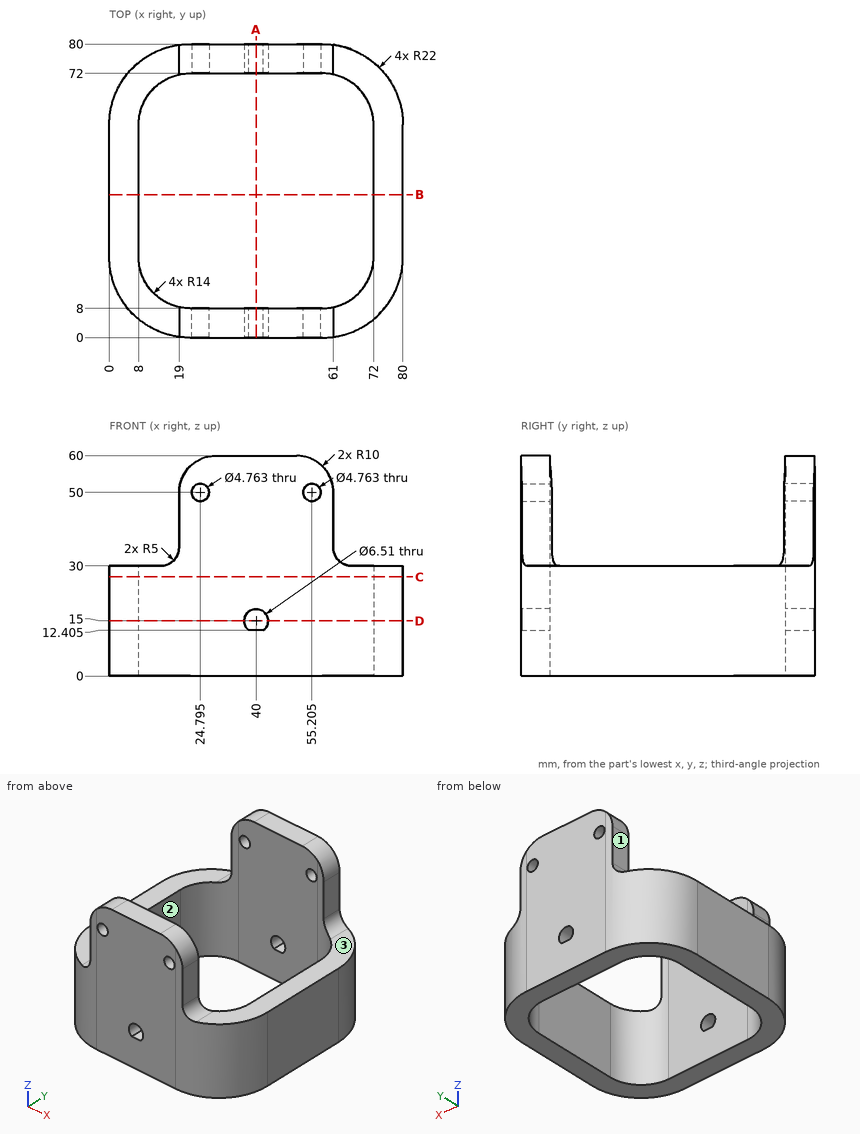
Check sheet for the drawn part. Datum: minimum x, y, z corner. Units: mm. A direction names the side the tool comes from. Coordinates: 2 decimals unless noted, no trailing zeros. Order: outer loops, then holes, each group sorted by start corner. A loop starts at its lowest first (then second) coordinate and runs counter-clockwise, first axis right, second up. Notation, with made-up numbers: (14.5, 77.25) - (23.5, 77.25) arc R5 cw to (23.5, 82.25) - close; hole circle Ø11 at (13.5, 8.25). An arc over 180 degrees is marked (long way). Return JSON: item names as keys, results as strings.
(1) Go/stop test with flat-tipped pins: pin 1 (2.5 mm diameter, centred on y = 75, z = 41, fed in from +X); pin 2 (11 mm diameter, centred on x = 9.5, y = 32, fed in from +Z); pin 3 (3 mm diameter, centred on y = 14, z = 21.5, fed in from -X); pin 4 (4.5 mm diameter, centred on x = 24.795, z = 50, fed in from -Y). Record where each tip stops, or that it passes through.
Filled sheet:
{"pin 1": "stops at x = 61", "pin 2": "stops at z = 30", "pin 3": "stops at x = 0.98", "pin 4": "passes through"}
(2) Section check D-D, the plane z = 15. Record the cut outline in (x, y) (1 decimal).
Filled sheet:
{"outline": "(0, 22) arc R22 ccw to (22, 0) - (36.7, 0) - (36.7, 8) - (22, 8) arc R14 cw to (8, 22) - (8, 58) arc R14 cw to (22, 72) - (36.7, 72) - (36.7, 80) - (22, 80) arc R22 ccw to (0, 58) - close; (43.3, 0) - (58, 0) arc R22 ccw to (80, 22) - (80, 58) arc R22 ccw to (58, 80) - (43.3, 80) - (43.3, 72) - (58, 72) arc R14 cw to (72, 58) - (72, 22) arc R14 cw to (58, 8) - (43.3, 8) - close"}
(3) Section check C-C, the plane z = 27. Record the cut outline in (x, y), and give its area (3 significant figures).
Filled sheet:
{"outline": "(0, 22) arc R22 ccw to (22, 0) - (58, 0) arc R22 ccw to (80, 22) - (80, 58) arc R22 ccw to (58, 80) - (22, 80) arc R22 ccw to (0, 58) - close; hole (8, 22) arc R14 ccw to (22, 8) - (58, 8) arc R14 ccw to (72, 22) - (72, 58) arc R14 ccw to (58, 72) - (22, 72) arc R14 ccw to (8, 58) - close", "area": "2,060 mm^2"}
(4) Thickness scan on line 1 along Z through (x, y) = (40, 2) (1 decimal); line 2 along X through (y, z) = (37.5, 5). Record the ranges inside material, lowest first.
Filled sheet:
{"line 1": "z = 0 to 12.4, 18.3 to 60", "line 2": "x = 0 to 8, 72 to 80"}
(5) Section check A-A, the plane x = 40. Record the cut outline in (y, z) (1 decimal).
Filled sheet:
{"outline": "(0, 0) - (8, 0) - (8, 12.4) - (0, 12.4) - close; (0, 18.3) - (8, 18.3) - (8, 60) - (0, 60) - close; (72, 0) - (80, 0) - (80, 12.4) - (72, 12.4) - close; (72, 18.3) - (80, 18.3) - (80, 60) - (72, 60) - close"}
(6) Section check B-B, the plane y = 39. Record the cut outline in (x, z).
Filled sheet:
{"outline": "(0, 0) - (8, 0) - (8, 30) - (0, 30) - close; (72, 0) - (80, 0) - (80, 30) - (72, 30) - close"}
(7) Access from +Z, -Z, +X, -X, +Y, -Y to the whole of each face (thin tool, end or side, straight path). Record for the marked faces 1, 2 and 3.
Filled sheet:
{"face 1": "+Z, -X, +Y, -Y", "face 2": "+Z, -Z", "face 3": "+Z, +X, +Y, -Y"}
